from build123d import *

# Parameters (mm, degrees)
F0_W     = 88.9
F0_H     = 431.8
F0_R     = 19.05
F1_DEPTH = 25.4


with BuildPart() as f1:
    # F0 (on Top) → F1 (new body)
    with BuildSketch(Plane.XY):
        Polygon((469.66731, 136.840239), (-444.73269, 136.840239), (-444.73269, -333.059761), (-444.73269, -371.159761), (469.66731, -371.159761), align=None)
        with Locations((-336.78269, -117.159761)):
            Rectangle(F0_W, F0_H, mode=Mode.SUBTRACT)
        with Locations((12.46731, 9.840239)):
            Circle(F0_R, mode=Mode.SUBTRACT)
        with Locations((361.71731, -117.159761)):
            Rectangle(F0_W, F0_H, mode=Mode.SUBTRACT)
    extrude(amount=F1_DEPTH)


solid = f1.part
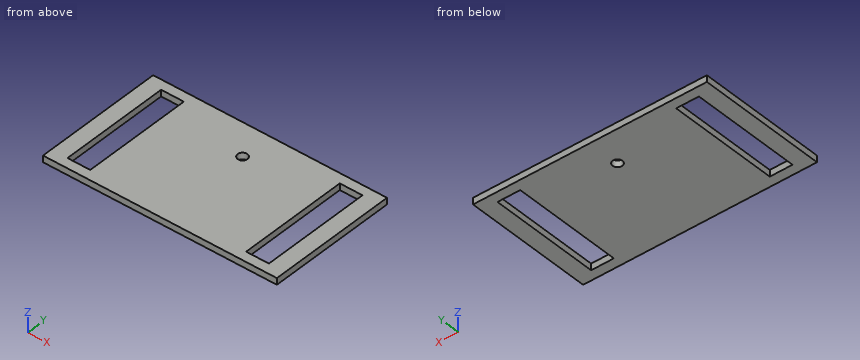
Design review of the part built by this model. Coordinates are the model's own, in mm. Give positions to 0.01 mm unless a question says otherwise; leave off trailing zeros. Order: outer loops, then holes, each group sorted by start corner. A loop starts at its lowest first (then second) coordinate and runs counter-clockwise, first axis right, second up. Notation, with made-up numbers: (2, 43) - (31, 43) arc R21 ccw to (31, 79) - close; hole circle Ø6 at (37, 33.25). An arc over 180 degrees is marked (long way). Use CSV: the item, a comma, the result in double quotes. Start each with the question number.
Q1. Take a section at B-B (y = 45). State the section outline as (x, z) points.
Q2. For line 1 (X direction, y = -182.5, z = 9.75); line 2 (X direction, y = 9, z = 22.5); line 3 (Y direction, x = -348, z = 9.25), list the stretches that pass through material, from the lowest coordinate up.
Q3. For P1, Ø6, axis at x = 92.5, y = -240, coming from the -Z side, flat-tipped, find the tip position at first contact; note if it passes through.
Q4. Take a section at A-A (x = 335). State the section outline as (y, z) points.
Q5. Take a section at C-C (z = 14). State the section outline as (x, y) points.
Calculated:
1,outline,"(-444.73, 0) - (-381.23, 0) - (-381.23, 25.4) - (-444.73, 25.4) - close; (-292.33, 0) - (317.27, 0) - (317.27, 25.4) - (-292.33, 25.4) - close; (406.17, 0) - (469.67, 0) - (469.67, 25.4) - (406.17, 25.4) - close"
2,line 1,"x = -444.73 to -381.23, -292.33 to 317.27, 406.17 to 469.67"
2,line 2,"x = -444.73 to -381.23, -292.33 to -6.56, 31.5 to 317.27, 406.17 to 469.67"
2,line 3,"y = -371.16 to -333.06, 98.74 to 136.84"
3,P1,"stops at z = 0"
4,outline,"(-371.16, 0) - (-333.06, 0) - (-333.06, 25.4) - (-371.16, 25.4) - close; (98.74, 0) - (136.84, 0) - (136.84, 25.4) - (98.74, 25.4) - close"
5,outline,"(-444.73, -371.16) - (469.67, -371.16) - (469.67, 136.84) - (-444.73, 136.84) - close; hole (-381.23, -333.06) - (-292.33, -333.06) - (-292.33, 98.74) - (-381.23, 98.74) - close; hole circle Ø38.1 at (12.47, 9.84); hole (317.27, -333.06) - (406.17, -333.06) - (406.17, 98.74) - (317.27, 98.74) - close"
